For this review, take the finished solid that the model builds, in its own axes (mm). A direction names the side the tool comes from. Give positions to 0.01 mm unless a question says otherwise; leave off trailing zeros. Order: outer loops, then holes, each group sorted by start corner. A loop starts at its lowest first (then second) coordinate and runs counter-clockwise, first axis right, second up. Notation, with made-up numbers: (-29, 15.5) -> (-18, 15.5) arc R22 ccw to (-18, 35.5) -> close; hole circle Ø5 at (28.25, 6). An arc over 180 degrees is marked (long way). One line per item, written item: value. Start each with the question number.
from build123d import *

# Parameters (mm, degrees)
F0_W      = 101.6
F0_H      = 50.8
F1_DEPTH  = 76.2
F2_W      = 31.3102314249
F2_H      = 69.1514285281
F2_W_2    = 30.7339653373
F3_DEPTH  = 45.72
F4_W      = 69.1514285281
F4_H      = 38.5872757655
F5_DEPTH  = 50.8
F6_W      = 15.24
F6_H      = 7.62
F7_DEPTH  = 10.16
F8_R      = 4.7199680321
F9_DEPTH  = 12.7
F10_R     = 1.635365768
F11_DEPTH = 1.524
F13_DEPTH = 1.524
F14_R     = 4.0060593356
F14_R_2   = 3.939714961
F15_DEPTH = 35.56


with BuildPart() as f1:
    # F0 (on Front) → F1 (new body)
    with BuildSketch(Plane.XZ):
        Rectangle(F0_W, F0_H)
    extrude(amount=-F1_DEPTH)

    # F2 (on face) → F3 (cut)
    with BuildSketch(Plane.XY.offset(25.4)):
        with Locations((-30.5790114217, 38.2802202366)):
            Rectangle(F2_W, F2_H)
        with Locations((31.561229378, 38.2802202366)):
            Rectangle(F2_W_2, F2_H)
    extrude(amount=-F3_DEPTH, mode=Mode.SUBTRACT)

    # F4 (on face) → F5 (cut)
    with BuildSketch(Plane(origin=(-14.9238957092, 0, 0), x_dir=(0, -1, 0), z_dir=(-1, 0, 0))):
        with Locations((-38.2802202366, -1.0263621172)):
            Rectangle(F4_W, F4_H)
    extrude(amount=-F5_DEPTH, mode=Mode.SUBTRACT)

    # F6 (on face) → F7 (cut)
    with BuildSketch(Plane.YZ.offset(50.8)):
        with Locations((36.6688001752, 0)):
            Rectangle(F6_W, F6_H)
    extrude(amount=-F7_DEPTH, mode=Mode.SUBTRACT)

    # F8 (on face) → F9 (cut)
    with BuildSketch(Plane(origin=(-50.8, 0, 0), x_dir=(0, -1, 0), z_dir=(-1, 0, 0))):
        with Locations((-38.1, 0)):
            Circle(F8_R)
    extrude(amount=-F9_DEPTH, mode=Mode.SUBTRACT)

    # F10 (on face) → F11 (cut)
    with BuildSketch(Plane.XZ):
        with BuildLine():
            ThreePointArc((0.8688539046, 16.0308553601), (2.2642224031, 17.0473777803), (2.7970019822, 18.6894852668))
            ThreePointArc((2.7970019822, 18.6894852668), (-1.728877271, 20.8881674789), (-0.6597016604, 15.9713951639))
            ThreePointArc((-0.6597016604, 15.9713951639), (0.108720026, 15.8945970679), (0.8688539046, 16.0308553601))
        make_face()
        with Locations((0, 18.6894852668)):
            Circle(F10_R, mode=Mode.SUBTRACT)
        with BuildLine():
            ThreePointArc((0.8688539046, 16.0308553601), (0.108720026, 15.8945970679), (-0.6597016604, 15.9713951639))
            Line((-0.6597016604, 15.9713951639), (-0.6597016604, 13.8239324768))
            Line((-0.6597016604, 13.8239324768), (-5.9159405627, 13.8239324768))
            Line((-5.9159405627, 13.8239324768), (-5.9159405627, 12.1085410579))
            Line((-5.9159405627, 12.1085410579), (-0.6597016604, 12.1085410579))
            ThreePointArc((-0.6597016604, 12.1085410579), (-0.0288400906, 3.1830218907), (-0.6597016604, -5.7424972765))
            ThreePointArc((-0.6597016604, -5.7424972765), (-6.2171832026, -9.0842868218), (-11.7746647447, -5.7424972765))
            Line((-11.7746647447, -5.7424972765), (-11.2480353564, -5.2158674225))
            ThreePointArc((-11.2480353564, -5.2158674225), (-12.6984808292, -4.2995334354), (-13.8811841607, -3.0566847418))
            ThreePointArc((-13.8811841607, -3.0566847418), (-13.5599978183, -5.3916725495), (-13.4072173387, -7.7436901629))
            Line((-13.4072173387, -7.7436901629), (-12.9332505167, -6.7430939525))
            ThreePointArc((-12.9332505167, -6.7430939525), (-8.0485977202, -9.9721592901), (-2.29532714, -11.0614588484))
            ThreePointArc((-2.29532714, -11.0614588484), (-0.6373782355, -12.0504785864), (0.8117884863, -13.3259668946))
            ThreePointArc((0.8117884863, -13.3259668946), (2.5191788748, -11.9655868759), (4.5508607291, -11.1667849123))
            ThreePointArc((4.5508607291, -11.1667849123), (10.5097684759, -10.3506913543), (15.2414478362, -6.6377678886))
            Line((15.2414478362, -6.6377678886), (15.7154146582, -8.112330921))
            ThreePointArc((15.7154146582, -8.112330921), (15.9275295852, -5.5845078314), (15.7154146582, -3.0566847418))
            ThreePointArc((15.7154146582, -3.0566847418), (15.0946685939, -4.1951955449), (14.4515028223, -5.3211930208))
            Line((14.4515028223, -5.3211930208), (14.4515028223, -5.8478228748))
            ThreePointArc((14.4515028223, -5.8478228748), (8.131944458, -9.5855520976), (1.8123860937, -5.8478228748))
            ThreePointArc((1.8123860937, -5.8478228748), (0.996836842, 3.1265252312), (1.1337217875, 12.1368141845))
            Line((1.1337217875, 12.1368141845), (6.5465644002, 12.1368141845))
            Line((6.5465644002, 12.1368141845), (6.5465644002, 13.683338151))
            Line((6.5465644002, 13.683338151), (0.8688539046, 13.683338151))
            Line((0.8688539046, 13.683338151), (0.8688539046, 16.0308553601))
        make_face()
        with BuildLine():
            ThreePointArc((0.8117884863, -8.7442873046), (2.1252827801, -8.2858759495), (2.9183086008, -9.4289062545))
            Line((2.9183086008, -9.4289062545), (0.8644514601, -11.9567289948))
            Line((0.8644514601, -11.9567289948), (-1.2947305804, -9.3235801905))
            ThreePointArc((-1.2947305804, -9.3235801905), (-0.4584292651, -8.2449949671), (0.8117884863, -8.7442873046))
        make_face(mode=Mode.SUBTRACT)
    extrude(amount=-F11_DEPTH, mode=Mode.SUBTRACT)

    # F12 (on face) → F13 (cut)
    with BuildSketch(Plane(origin=(0, 76.2, 0), x_dir=(-1, 0, 0), z_dir=(0, 1, 0))):
        with BuildLine():
            Line((14.2345046625, 20.9841318429), (0, 3.4671491012))
            Line((0, 3.4671491012), (-13.7768853456, 20.7474157214))
            Line((-13.7768853456, 20.7474157214), (-15.1745732773, 19.6330934249))
            Line((-15.1745732773, 19.6330934249), (-1.1224173427, 2.0075565166))
            Line((-1.1224173427, 2.0075565166), (-11.2962679055, -10.512384918))
            ThreePointArc((-11.2962679055, -10.512384918), (-16.9222450094, -10.615651057), (-22.3775655031, -9.2366077006))
            ThreePointArc((-22.3775655031, -9.2366077006), (-24.377281906, -10.3599397452), (-23.4822407365, -12.4717261642))
            ThreePointArc((-23.4822407365, -12.4717261642), (-18.0084948263, -14.6788471986), (-12.1198734269, -15.0756035))
            Line((-12.1198734269, -15.0756035), (0, 0))
            Line((0, 0), (12.4196829274, -15.2334133163))
            ThreePointArc((12.4196829274, -15.2334133163), (17.9436167829, -14.9653793634), (23.2297126204, -13.3396862075))
            ThreePointArc((23.2297126204, -13.3396862075), (24.9682567409, -11.1020125383), (22.835187614, -9.2366077006))
            ThreePointArc((22.835187614, -9.2366077006), (17.49741351, -10.7969617685), (11.9462516159, -11.1303366721))
            Line((11.9462516159, -11.1303366721), (1.0416547929, 2.0300080541))
            Line((1.0416547929, 2.0300080541), (15.5652534262, 19.9027498628))
            Line((15.5652534262, 19.9027498628), (14.2345046625, 20.9841318429))
        make_face()
    extrude(amount=-F13_DEPTH, mode=Mode.SUBTRACT)

    # F14 (on face) → F15 (join)
    with BuildSketch(Plane.XY.offset(-20.32)):
        with Locations((-26.4782663435, 55.7343438268)):
            Circle(F14_R)
        with Locations((26.2298732996, 13.9785446227)):
            Circle(F14_R_2)
    extrude(amount=F15_DEPTH)


solid = f1.part
Q1. For pin 1 Ø4 at (x, y) = (-25, 57) entering from +Z; pin 2 Ø8 at (x, y) = (-19.5, 39.5) entering from +Z, all flat-tipped, find the tip position at first contact; note any pin that passes through.
Q2. Mouldability with a two-part tool opening along Y and no side actions: class faces 1 (the cylindrical face through (24.366, 75.449, -10.327)), 2 (the flat face through (2, 74.676, -1)), 3 (the flat face through (0, 0, 19)), 4 (the flat face through (46.928, 38, 8)) as pulls with the +Y half, pulls with the -Y half, needs draft (parallel to the pull), parting line crosses it, or undercut.
Q3. Take a section at B-B (y = 38.1). State the section outline as (x, z) points, and give its area (3 significant figures).
Q4. Take a section at A-A (z = -19). State the section outline as (x, y) points.
Q5. Take a section at D-D (x = 9). State the section outline as (y, z) points.
Q6. Take a section at C-C (x = 40). State the section outline as (y, z) points.
Q7. For line 1 along X through (y, z) = (24.5, 17); line 2 along Y through (x, z) = (-38, -10.5); line 3 along Z through (x, y) = (1.5, 45), list the stretches that pass through material, from the lowest coordinate up.
Q8. For faces 5 (the cylindrical face through (-27, 59.706, -2.789)), 6 (the flat face through (-6.57, 75.45, -4.64)), 7 (the flat face through (0, 72.856, 3)), 8 (the cylindrical face through (-0.659, 0.751, -12.035)), list the 3-axis set-ups (+Z, -Z, +X, -X, +Y, -Y) from which the entire face can be reached by the end or side of a thin tool; tool diameter is ignored.
Answers below:
1. pin 1: stops at z = 15.24
1. pin 2: stops at z = -20.32
2. face 1: needs draft
2. face 2: pulls with the +Y half
2. face 3: pulls with the -Y half
2. face 4: undercut
3. outline: (-50.8, -25.4) -> (50.8, -25.4) -> (50.8, -3.81) -> (46.93, -3.81) -> (46.93, -20.32) -> (-46.23, -20.32) -> (-46.23, -4.72) -> (-50.8, -4.72) -> close; (-50.8, 4.72) -> (-46.23, 4.72) -> (-46.23, 25.4) -> (-50.8, 25.4) -> close; (-14.92, 18.27) -> (16.19, 18.27) -> (16.19, 25.4) -> (-14.92, 25.4) -> close; (46.93, 3.81) -> (50.8, 3.81) -> (50.8, 25.4) -> (46.93, 25.4) -> close
3. area: 1,050 mm²
4. outline: (-50.8, 0) -> (50.8, 0) -> (50.8, 76.2) -> (-50.8, 76.2) -> close; circle Ø8.01 at (-26.48, 55.73); circle Ø7.88 at (26.23, 13.98); hole (-46.23, 3.7) -> (46.93, 3.7) -> (46.93, 72.86) -> (-46.23, 72.86) -> close
5. outline: (0, -25.4) -> (76.2, -25.4) -> (76.2, -11.19) -> (74.68, -11.19) -> (74.68, -7.69) -> (76.2, -7.69) -> (76.2, 11.89) -> (74.68, 11.89) -> (74.68, 14.76) -> (76.2, 14.76) -> (76.2, 25.4) -> (0, 25.4) -> (0, -9.53) -> (1.52, -9.53) -> (1.52, -10.87) -> (0, -10.87) -> close; hole (3.7, -20.32) -> (72.86, -20.32) -> (72.86, 18.27) -> (3.7, 18.27) -> close
6. outline: (0, -25.4) -> (76.2, -25.4) -> (76.2, 25.4) -> (72.86, 25.4) -> (72.86, -20.32) -> (3.7, -20.32) -> (3.7, 25.4) -> (0, 25.4) -> close
7. line 1: x = -50.8 to -46.23, 46.93 to 50.8
7. line 2: y = 0 to 3.7, 72.86 to 76.2
7. line 3: z = -25.4 to -20.32, 18.27 to 25.4
8. face 5: +Z
8. face 6: +Y
8. face 7: none
8. face 8: -Y
